Geometry: final body of the model. Coordinates: model frame, mm. A direction names the side the tool comes from. Give positions to 0.01 mm unless a question says otherwise; leave off trailing zeros. Order: outer loops, then holes, each group sorted by start corner. A loop starts at its lowest first (then second) coordinate and runs counter-clockwise, first axis right, second up. Notation, with made-up numbers: (-18.75, 56) - (19.25, 56) arc R14 ccw to (19.25, 69) - close; hole circle Ø8 at (34, -24.75). An arc over 180 degrees is marked (long way). Use one line per item in the form item = value.
from build123d import *

# Parameters (mm, degrees)
PAD_DEPTH = 3.175
FILLET_R  = 1.016


with BuildPart() as part:
    # Sketch → Pad (new body)
    with BuildSketch(Plane.XY):
        with BuildLine():
            Line((-16.51, 3.302), (-17.762531, -7.32262))
            ThreePointArc((-17.762531, -7.32262), (-15.994846, -10.045244), (-12.994271, -8.806719))
            Line((-12.994271, -8.806719), (-9.525, -2.241526))
            ThreePointArc((-9.525, -2.241526), (-5.441505, -2.962411), (-2.54, 0))
            Line((-2.54, 0), (2.54, 0))
            ThreePointArc((2.54, 0), (5.441505, -2.962411), (9.525, -2.241526))
            Line((9.525, -2.241526), (12.994271, -8.806719))
            ThreePointArc((12.994271, -8.806719), (15.994846, -10.045244), (17.762531, -7.32262))
            Line((17.762531, -7.32262), (16.51, 3.302))
            Line((16.51, 3.302), (16.888459, 11.322248))
            ThreePointArc((16.888459, 11.322248), (15.501948, 13.532684), (12.946847, 13.003634))
            Line((12.946847, 13.003634), (9.525, 9.398))
            Line((9.525, 9.398), (7.473462, 10.999677))
            ThreePointArc((7.473462, 10.999677), (6.223, 11.43), (4.972538, 10.999677))
            Line((4.972538, 10.999677), (2.921, 9.398))
            Line((2.921, 9.398), (-2.921, 9.398))
            Line((-2.921, 9.398), (-4.972538, 10.999677))
            ThreePointArc((-4.972538, 10.999677), (-6.223, 11.43), (-7.473462, 10.999677))
            Line((-7.473462, 10.999677), (-9.525, 9.398))
            Line((-9.525, 9.398), (-12.946847, 13.003634))
            ThreePointArc((-12.946847, 13.003634), (-15.501948, 13.532684), (-16.888459, 11.322248))
            Line((-16.888459, 11.322248), (-16.51, 3.302))
        make_face()
    extrude(amount=PAD_DEPTH)

    # Fillet
    fillet_edges = [part.edges().sort_by_distance(p)[0] for p in [
        (-9.525, 9.398, 1.5875),
        (9.525, 9.398, 1.5875),
    ]]
    fillet(fillet_edges, radius=FILLET_R)


solid = part.part
(1) Contact query for flat-ended pins moving along their axis: pin 1 Ø1 at (y, z) = (0.5, 2) entering from +X; pin 2 Ø1.6 at (x, z) = (0, 1) entering from -Y; pin 3 Ø1.6 at (x, z) = (0, 2) entering from +Y. Output: stop coordinate, or through.
Computed values:
pin_1 = 16.9
pin_2 = 0
pin_3 = 9.4
(2) Cut plane D-D on x = -2. Output: boundary loops of the cut face in (y, z) (3 decimals), plus the area to 3 significant figures.
Computed values:
outline = (0, 0) - (9.398, 0) - (9.398, 3.175) - (0, 3.175) - close
area = 29.8 mm²
(3) Cut plane C-C on y = -1. Output: boundary loops of the cut face in (x, z) (3 decimals).
Computed values:
outline = (-17.017, 0) - (-2.978, 0) - (-2.978, 3.175) - (-17.017, 3.175) - close; (2.978, 0) - (17.017, 0) - (17.017, 3.175) - (2.978, 3.175) - close
(4) Pull-direction query (X, two-part tool) for faces 4 (the face through (-17.127, -1.936, 1.565)), 5 (the face through (9.509, 9.754, 1.61)), 6 (the face through (16.7, 7.3, 1.6)); classes: released by +X, released by -X, zero draft, split by the parting line, or undercut.
Computed values:
face_4 = released by -X
face_5 = undercut
face_6 = released by +X
(5) Cut plane A-A on y = 10.5. Output: boundary loops of the cut face in (x, z) (3 decimals).
Computed values:
outline = (-16.85, 0) - (-10.571, 0) - (-10.571, 3.175) - (-16.85, 3.175) - close; (-8.113, 0) - (-4.333, 0) - (-4.333, 3.175) - (-8.113, 3.175) - close; (4.333, 0) - (8.113, 0) - (8.113, 3.175) - (4.333, 3.175) - close; (10.571, 0) - (16.85, 0) - (16.85, 3.175) - (10.571, 3.175) - close
(6) Ray query, line 1 along X through (y, z) = (-4.5, 3); line 2 along Y through (x, z) = (-1.5, 0.8); line 3 along X through (y, z) = (10.5, 1). Return the intervals inside material, ascending.
Computed values:
line_1 = -17.43 to -10.72, 10.72 to 17.43
line_2 = 0 to 9.4
line_3 = -16.85 to -10.57, -8.11 to -4.33, 4.33 to 8.11, 10.57 to 16.85
(7) Cut plane B-B on z = 2.75. Output: boundary loops of the cut face in (x, y) (3 decimals), plus the area to 3 significant figures.
Computed values:
outline = (-17.763, -7.323) arc R2.54 ccw to (-12.994, -8.807) - (-9.525, -2.242) arc R4.445 ccw to (-2.54, 0) - (2.54, 0) arc R4.445 ccw to (9.525, -2.242) - (12.994, -8.807) arc R2.54 ccw to (17.763, -7.323) - (16.51, 3.302) - (16.888, 11.322) arc R2.286 ccw to (12.947, 13.004) - (10.16, 10.067) arc R1.016 cw to (8.798, 9.966) - (7.473, 11) arc R2.032 ccw to (4.973, 11) - (2.921, 9.398) - (-2.921, 9.398) - (-4.973, 11) arc R2.032 ccw to (-7.473, 11) - (-8.798, 9.966) arc R1.016 cw to (-10.16, 10.067) - (-12.947, 13.004) arc R2.286 ccw to (-16.888, 11.322) - (-16.51, 3.302) - close
area = 533 mm²
(8) Reachability of faces 1 (the face through (11.235, -5.478, 1.565)), 2 (the face through (11.573, 11.556, 1.565)), 3 (the face through (0, 2, 0)) from +Z, -Z, +X, -X, +Y, -Y: full face, straight path, thin tool, end or side. Return the list, or none.
Computed values:
face_1 = +Z, -Z, -Y
face_2 = +Z, -Z, +Y
face_3 = -Z, +X, -X, +Y, -Y
